Build history of the part. All positions in model axes, mm. A direction names the side the tool comes from. Round coordinates to 2 decimals unless told otherwise and drop trailing zeros. Write each loop counter-clockwise with the first axis right and the second up, starting at its lowest first coordinate (ties: lowest second). Pieces come first, ordered by that corner, then holes. Notation, with made-up numbers: (-39, 83.25) -> (-13, 83.25) arc R9 cw to (-13, 87.25) -> close; hole circle Ø5 at (-26, -15). An arc over 180 degrees is marked (long way). Return JSON: item names as keys, results as strings.
from build123d import *

# Parameters (mm, degrees)
F0_R     = 4.7625
F0_R_2   = 8
F1_DEPTH = 4.83


with BuildPart() as f1:
    # F0 (on Top) → F1 (new body)
    with BuildSketch(Plane.XY):
        with BuildLine():
            ThreePointArc((2.5, 13.80407), (2.784562, 14.962445), (3.573466, 15.857117))
            ThreePointArc((3.573466, 15.857117), (0, 27.2625), (-3.573466, 15.857117))
            ThreePointArc((-3.573466, 15.857117), (-2.784562, 14.962445), (-2.5, 13.80407))
            Line((-2.5, 13.80407), (-2.5, 12))
            ThreePointArc((-2.5, 12), (-2.919874, 10.61325), (-4.038462, 9.692308))
            ThreePointArc((-4.038462, 9.692308), (-9.093267, 5.25), (-10.413015, -1.348744))
            ThreePointArc((-10.413015, -1.348744), (-10.651281, -2.777939), (-11.642305, -3.834936))
            Line((-11.642305, -3.834936), (-13.204675, -4.736972))
            ThreePointArc((-13.204675, -4.736972), (-14.350139, -5.069722), (-15.5194, -4.833846))
            ThreePointArc((-15.5194, -4.833846), (-23.610018, -13.63125), (-11.945933, -11.023271))
            ThreePointArc((-11.945933, -11.023271), (-11.565577, -9.892724), (-10.704675, -9.067099))
            Line((-10.704675, -9.067099), (-9.142305, -8.165064))
            ThreePointArc((-9.142305, -8.165064), (-7.731407, -7.83531), (-6.374554, -8.343564))
            ThreePointArc((-6.374554, -8.343564), (0, -10.5), (6.374554, -8.343564))
            ThreePointArc((6.374554, -8.343564), (7.731407, -7.83531), (9.142305, -8.165064))
            Line((9.142305, -8.165064), (10.704675, -9.067099))
            ThreePointArc((10.704675, -9.067099), (11.565577, -9.892724), (11.945933, -11.023271))
            ThreePointArc((11.945933, -11.023271), (23.610018, -13.63125), (15.5194, -4.833846))
            ThreePointArc((15.5194, -4.833846), (14.350139, -5.069722), (13.204675, -4.736972))
            Line((13.204675, -4.736972), (11.642305, -3.834936))
            ThreePointArc((11.642305, -3.834936), (10.651281, -2.777939), (10.413015, -1.348744))
            ThreePointArc((10.413015, -1.348744), (9.093267, 5.25), (4.038462, 9.692308))
            ThreePointArc((4.038462, 9.692308), (2.919874, 10.61325), (2.5, 12))
            Line((2.5, 12), (2.5, 13.80407))
        make_face()
        with Locations((-18.186533, -10.5)):
            Circle(F0_R, mode=Mode.SUBTRACT)
        with Locations((18.186533, -10.5)):
            Circle(F0_R, mode=Mode.SUBTRACT)
        Circle(F0_R_2, mode=Mode.SUBTRACT)
        with Locations((0, 21)):
            Circle(F0_R, mode=Mode.SUBTRACT)
    extrude(amount=F1_DEPTH)


solid = f1.part
Q1. Saw through at B-B on x = 0. List the corners of the cut face in (y, z), then the cut area to 3 significant figures.
Verdict:
{"outline": "(-10.5, 0) -> (-8, 0) -> (-8, 4.83) -> (-10.5, 4.83) -> close; (8, 0) -> (16.24, 0) -> (16.24, 4.83) -> (8, 4.83) -> close; (25.76, 0) -> (27.26, 0) -> (27.26, 4.83) -> (25.76, 4.83) -> close", "area": "59.1 mm²"}
Q2. Saw through at C-C on x = -19. List the corners of the cut face in (y, z), then the cut area to 3 significant figures.
Verdict:
{"outline": "(-16.71, 0) -> (-15.19, 0) -> (-15.19, 4.83) -> (-16.71, 4.83) -> close; (-5.81, 0) -> (-4.29, 0) -> (-4.29, 4.83) -> (-5.81, 4.83) -> close", "area": "14.7 mm²"}
Q3. Saw through at A-A on y = 0. List the corners of the cut face in (x, z), then the cut area to 4 significant figures.
Verdict:
{"outline": "(-10.5, 0) -> (-8, 0) -> (-8, 4.83) -> (-10.5, 4.83) -> close; (8, 0) -> (10.5, 0) -> (10.5, 4.83) -> (8, 4.83) -> close", "area": "24.15 mm²"}
Q4. 3-axis set-ups, long thin cutter, end or side, ignore diameter. For faces 4 (the flat face through (12.43, -4.29, 2.38)), 5 (the cylindrical face through (2.78, 14.95, 2.38)), 6 (the cylindrical face through (-9.045, 5.333, 2.381)), 7 (the cylindrical face through (11.556, -9.879, 2.381)): which of +Z, -Z, +X, -X, +Y, -Y reach the whole face in a straight line?
Verdict:
{"face 4": "+Z, -Z, +Y", "face 5": "+Z, -Z, +X", "face 6": "+Z, -Z, -X", "face 7": "+Z, -Z, -Y"}
Q5. Wall check: L1, parallel to Y at x = 3, z = 4.3; L2, parallel to Y at x = -1.5, z = 4.25; L3, parallel to X at y = -14, z = 3.6. Give the ranges that are in metal, low to high.
Verdict:
{"L1": "y = -10.06 to -7.42, 7.42 to 10.5, 15.3 to 17.3, 24.7 to 26.5", "L2": "y = -10.39 to -7.86, 7.86 to 16.48, 25.52 to 27.08", "L3": "x = -23.38 to -21.42, -14.96 to -12.99, 12.99 to 14.96, 21.42 to 23.38"}
Q6. Pin check, flat tips, straight feed: pin 1 Ø2 at (y, z) = (12.5, 2) entering from +X; pin 2 Ø1 at (x, z) = (2.5, 1) entering from -Y; pin 3 Ø11 at (x, y) = (18.19, -10.5) entering from +Z; pin 4 Ø2 at (y, z) = (13, 1.5) entering from -X. Stop position of each tip, or through.
Verdict:
{"pin 1": "stops at x = 2.55", "pin 2": "stops at y = -10.31", "pin 3": "stops at z = 4.83", "pin 4": "stops at x = -2.51"}
Q7. Saw through at D-D on z = 2.45. List the corners of the cut face in (x, y) (1 decimal), then the cut area to 3 significant figures.
Verdict:
{"outline": "(-15.5, -4.8) arc R6.3 ccw (long way) to (-11.9, -11) arc R2.5 cw to (-10.7, -9.1) -> (-9.1, -8.2) arc R2.5 cw to (-6.4, -8.3) arc R10.5 ccw to (6.4, -8.3) arc R2.5 cw to (9.1, -8.2) -> (10.7, -9.1) arc R2.5 cw to (11.9, -11) arc R6.3 ccw (long way) to (15.5, -4.8) arc R2.5 cw to (13.2, -4.7) -> (11.6, -3.8) arc R2.5 cw to (10.4, -1.3) arc R10.5 ccw to (4, 9.7) arc R2.5 cw to (2.5, 12) -> (2.5, 13.8) arc R2.5 cw to (3.6, 15.9) arc R6.3 ccw (long way) to (-3.6, 15.9) arc R2.5 cw to (-2.5, 13.8) -> (-2.5, 12) arc R2.5 cw to (-4, 9.7) arc R10.5 ccw to (-10.4, -1.3) arc R2.5 cw to (-11.6, -3.8) -> (-13.2, -4.7) arc R2.5 cw to start; hole circle Ø9.5 at (-18.2, -10.5); hole circle Ø16 at (0, 0); hole circle Ø9.5 at (0, 21); hole circle Ø9.5 at (18.2, -10.5)", "area": "374 mm²"}
Q8. Two-plate mould, pull along X, no slides. Class faces 1 (the flat face through (-7.4, 3.7, 4.83)), 2 (the cylindrical face through (-2.91, 10.63, 2.38)), 3 (the flat face through (9.91, -8.61, 2.38)): +X half, -X half, draft (parallel to the pull), parting line (faces both ways), or undercut.
Verdict:
{"face 1": "draft", "face 2": "-X half", "face 3": "undercut"}
